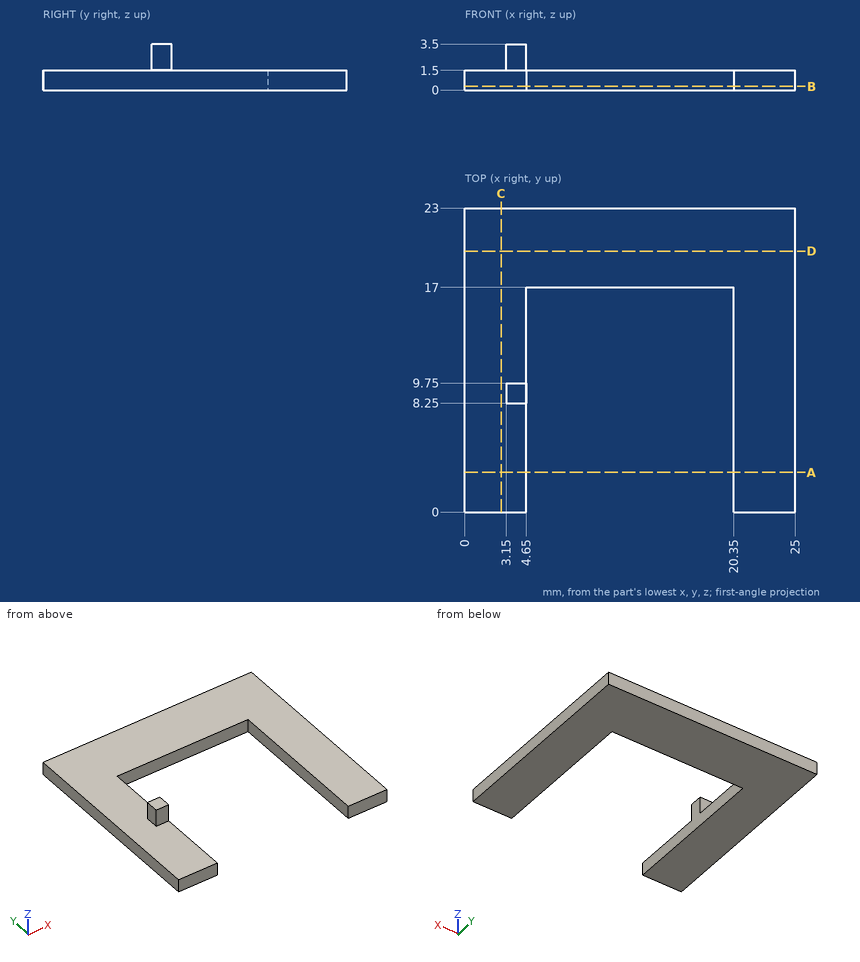
Input: dimensioned drawing with shaded views. Units: mm. Origin: part minimum x, y, z. Coordinates: 2 decimals unless noted, no trailing zeros. Loops run counter-clockwise (first coordinate to the right, second up) from the corner with the lowest first, then second, coordinate; pieces in that order, holes last. Notation, with made-up numbers: M 54.5,66.25 L 111.5,66.25 A6 cw 111.5,71.25 Z; hole C -24.75,80.5 d11. An arc over 180 degrees is marked long. Use a Markdown table: item, result. Add a question column.
1) Section B-B, the plane z = 0.3. Return the cut outline in (x, y), plus the area to 3 significant figures.
2) Pin query (flat end, axial travel): P1, Ø5, axis at x = 19, y = 4, coming from the +Z side; P2, Ø1.2, axis at x = 11, z = 1, coming from the -Y side; P3, Ø0.8, axis at y = 9.5, z = 2, coming from the -X side. Return the tip coordinate at first contact, or that it passes through.
3) Section C-C, the plane x = 2.75. Return the cut outline in (y, z), plus the area to 3 significant figures.
4) Section A-A, the plane y = 3. Return the cut outline in (x, z), plus the area to 4 significant figures.
5) Line query: L1, parallel to X at y = 3.25, z = 1.4; L2, parallel to Z at x = 20.5, y = 8.75; L3, parallel to Y at x = 19.25, z = 0.25. Output: solid intervals per line, ascending. Write a range as from..to.
6) Section D-D, the plane y = 19.75. Return the cut outline in (x, z).
Answer below:
| question | item | result |
|---|---|---|
| 1 | outline | M 0,0 L 4.65,0 L 4.65,17 L 20.35,17 L 20.35,0 L 25,0 L 25,23 L 0,23 Z |
| 1 | area | 308 mm2 |
| 2 | P1 | z = 1.5 |
| 2 | P2 | y = 17 |
| 2 | P3 | x = 3.15 |
| 3 | outline | M 0,0 L 23,0 L 23,1.5 L 0,1.5 Z |
| 3 | area | 34.5 mm2 |
| 4 | outline | M 0,0 L 4.65,0 L 4.65,1.5 L 0,1.5 Z; M 20.35,0 L 25,0 L 25,1.5 L 20.35,1.5 Z |
| 4 | area | 13.95 mm2 |
| 5 | L1 | 0..4.65, 20.35..25 |
| 5 | L2 | 0..1.5 |
| 5 | L3 | 17..23 |
| 6 | outline | M 0,0 L 25,0 L 25,1.5 L 0,1.5 Z |
